Part print with two shaded views. Sizes in mm from the minimum x, y, z corner. Coordinates: 2 decimals unless noted, no trailing zeros. Loops run counter-clockwise (first coordinate to the right, second up) from the corner with the lowest first, then second, coordinate; pieces in that order, holes last.
(1) Slice it at C-C (z = 189). Give the cut face in (x, y), and give its area (3 significant figures).
(2) Slice it at B-B (z = 139.5). Give the cut face in (x, y).
(3) Flat gauge pins, fed straight in: P1, Ø1.9, axis at y = 3.5, z = 3, coming from the +X side; P2, Ø3, axis at x = 121, y = 2, coming from the -Z side. Where does each tip first touch, or does it go through?
(4) Slice it at D-D (y = 3.5). Give the number of separate pieces and of enclosed holes in the cut face, and give its area (3 significant figures).
(5) Wall check: L1, parallel to X at y = 3, z = 90; L2, parallel to X at y = 3, z = 236.5; L3, parallel to Z at x = 90, y = 4 (1 decimal). Give the ranges that are in metal, low to high.
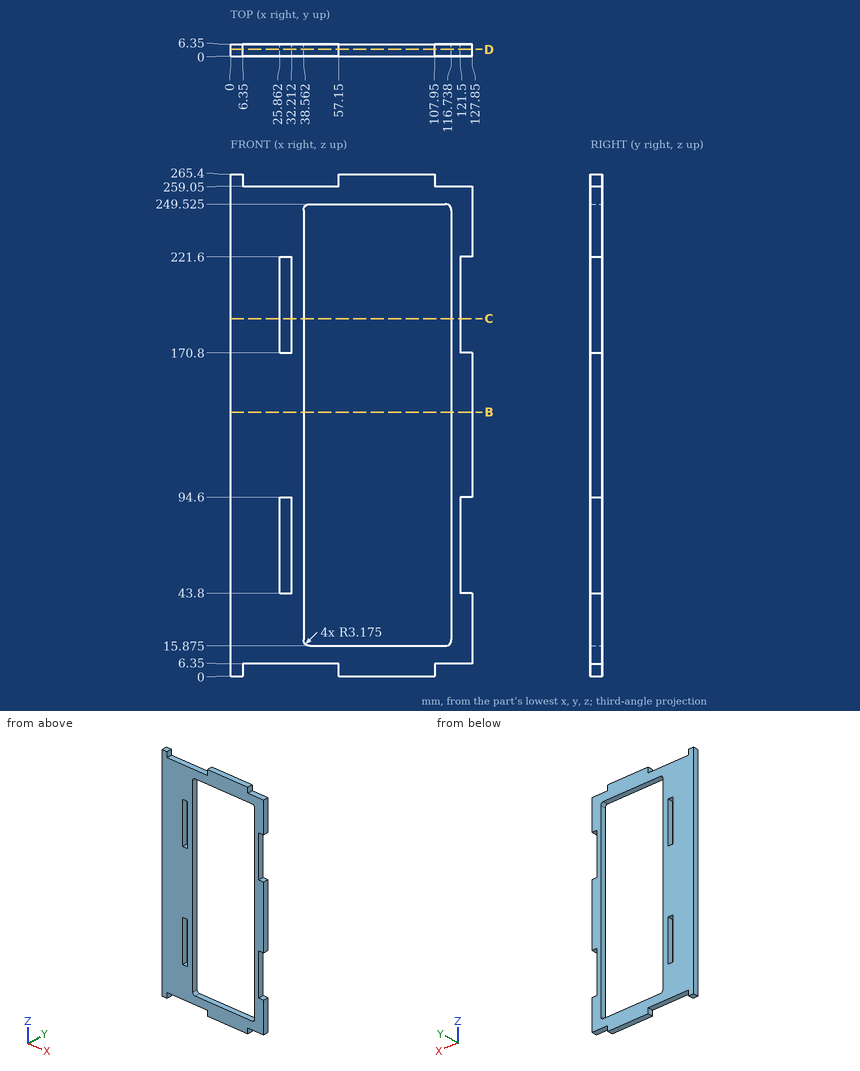
Response values:
1. outline: (0, 0) - (25.86, 0) - (25.86, 6.35) - (0, 6.35) - close; (32.21, 0) - (38.56, 0) - (38.56, 6.35) - (32.21, 6.35) - close; (116.74, 0) - (121.5, 0) - (121.5, 6.35) - (116.74, 6.35) - close
1. area: 235 mm2
2. outline: (0, 0) - (38.56, 0) - (38.56, 6.35) - (0, 6.35) - close; (116.74, 0) - (127.85, 0) - (127.85, 6.35) - (116.74, 6.35) - close
3. P1: stops at x = 107.95
3. P2: stops at z = 6.35
4. separate pieces: 1
4. enclosed holes: 3
4. area: 13,500 mm2
5. L1: x = 0 to 25.86, 32.21 to 38.56, 116.74 to 121.5
5. L2: x = 0 to 38.56, 116.74 to 127.85
5. L3: z = 0 to 15.9, 249.5 to 265.4
